Read the model definition and answer for the solid it produces. Units are mm, in the model's axes. A direction names the side the tool comes from. Coordinates: 2 decimals unless noted, no trailing zeros. Loops run counter-clockwise (first coordinate to the right, second up) from the corner with the lowest first, then second, coordinate; pieces in that order, holes last.
from build123d import *

# Parameters (mm, degrees)
SKETCH_1_R           = 2
EXTRUDE_1_DEPTH      = 16
EXTRUDE_2_DEPTH      = 3.175
SKETCH_4_R           = 3.15
CUT_EXTRUDE_6_DEPTH  = 2.775
FILLET_3_R           = 0.6
SKETCH_7_R           = 3.175
EXTRUDE_3_DEPTH      = 1.4
CUT_EXTRUDE_10_DEPTH = 10
FILLET_4_R           = 0.3
CUT_EXTRUDE_11_REACH = 18
FILLET_5_R           = 1


with BuildPart() as part:
    # 草图1 → 凸台-拉伸1 (new body)
    with BuildSketch(Plane(origin=(0, 0, 0), x_dir=(1, 0, 0), z_dir=(0, 1, 0))):
        Circle(SKETCH_1_R)
    extrude(amount=EXTRUDE_1_DEPTH)

    # 草图2 → 凸台-拉伸2 (add)
    with BuildSketch(Plane.XY):
        with BuildLine():
            Line((3.175, 16), (1.070738578, 21.991208882))
            ThreePointArc((1.070738578, 21.991208882), (-6.846541908, 23.101880092), (-3.175, 16))
            Line((-3.175, 16), (3.175, 16))
        make_face()
    extrude(amount=EXTRUDE_2_DEPTH)

    # 草图4 → 切除-拉伸6 (cut)
    with BuildSketch(Plane(origin=(0, 0, 0), x_dir=(-1, 0, 0), z_dir=(0, 0, -1))):
        with Locations((3.175, 20.5)):
            Circle(SKETCH_4_R)
    extrude(amount=-CUT_EXTRUDE_6_DEPTH, mode=Mode.SUBTRACT)

    # 圆角3
    fillet_3_edges = [part.edges().sort_by_distance(p)[0] for p in [
        (-2, 0, 0),
    ]]
    fillet(fillet_3_edges, radius=FILLET_3_R)

    # 草图7 → 凸台-拉伸3 (add)
    with BuildSketch(Plane(origin=(0, 16, 0), x_dir=(1, 0, 0), z_dir=(0, 1, 0))):
        Circle(SKETCH_7_R)
    extrude(amount=-EXTRUDE_3_DEPTH)

    # 草图11 → 切除-拉伸10 (cut, through all)
    with BuildSketch(Plane.XZ.offset(-16)):
        with BuildLine():
            Line((3.175, 3.175), (3.50604204, 0.275))
            Line((3.50604204, 0.275), (3.175, 0))
            ThreePointArc((3.175, 0), (2.24506403, 2.24506403), (0, 3.175))
            Line((0, 3.175), (3.175, 3.175))
        make_face()
    extrude(amount=-CUT_EXTRUDE_10_DEPTH, mode=Mode.SUBTRACT)

    # 草图12 → 旋转1 (revolve)
    with BuildSketch(Plane(origin=(0, 20.5, 0), x_dir=(-1, 0, 0), z_dir=(0, -1, 0))):
        with BuildLine():
            Line((3.8375, -3.175), (3.8375, -3.475))
            ThreePointArc((3.8375, -3.475), (5.765394552, -3.441974066), (7.675, -3.175))
            Line((7.675, -3.175), (3.8375, -3.175))
        make_face()
    revolve(axis=Axis((-3.8375, 20.5, 3.175), (0, 0, 1)))

    # 圆角4
    fillet_4_edges = [part.edges().sort_by_distance(p)[0] for p in [
        (-0.025, 20.5, 0),
    ]]
    fillet(fillet_4_edges, radius=FILLET_4_R)

    # 草图13 → 切除-拉伸11 (cut, up to next)
    with BuildSketch(Plane(origin=(0, 16, 0), x_dir=(1, 0, 0), z_dir=(0, 1, 0)), mode=Mode.PRIVATE) as cut_extrude_11_sk1:
        with BuildLine():
            Line((-1.4, 0), (1.4, 0))
            ThreePointArc((1.4, 0), (0, 1.4), (-1.4, 0))
        make_face()
    cut_extrude_11_tool1 = extrude(cut_extrude_11_sk1.sketch, amount=-CUT_EXTRUDE_11_REACH, mode=Mode.PRIVATE) & part.part
    add(cut_extrude_11_tool1.solids().sort_by_distance((0, 16, -0.594178))[0], mode=Mode.SUBTRACT)

    # 圆角5
    fillet_5_edges = [part.edges().sort_by_distance(p)[0] for p in [
        (0, 16, -1.4),
    ]]
    fillet(fillet_5_edges, radius=FILLET_5_R)


solid = part.part
Q1. Flat-ended cylindrical pins translate along their axes: pin 1 Ø2.5 at (x, y) = (-5.5, 18.5) entering from +Z; pin 2 Ø1 at (x, z) = (-5.5, 1) entering from -Y; pin 3 Ø1.6 at (x, z) = (1, -1) entering from +Y. Find the tip coordinate at first contact, or state that the pin passes through.
Findings below:
pin 1: stops at z = 3.48
pin 2: stops at y = 16.39
pin 3: stops at y = 15.98
Q2. Straight lines are drawn through the part: probe 1 along Y at (x, z) = (-2, -1.25); probe 2 along Y at (x, z) = (-5, 0.25); probe 3 along Z at (x, y) = (0, 1.5). For each, find the intervals that lie inside material, in ascending order.
Findings below:
probe 1: y = 14.6 to 16
probe 2: y = 16.39 to 17.93, 23.07 to 24.61
probe 3: z = -2 to -1.4, 0 to 2
Q3. A cutting plane is placed at A-A (y = 12.5). Give the vertices of the cut face in (x, z).
Findings below:
outline: circle Ø4 at (0, 0); hole (-1.4, 0) arc R1.4 ccw to (1.4, 0) - close
Q4. Which of the six approach directions +Z, -Z, +X, -X, +Y, -Y give full straight-line access (tool end or side, diameter ignored) to faces 4 (the face through (0, 7.6, -1.4)), 5 (the face through (-2.4, 24.3, 3.175)), 6 (the face through (0, 8, 2))?
Findings below:
face 4: +Y, -Y
face 5: +Z, +Y
face 6: -Y
Q5. Determine the mould class of faces 1 (the face through (1, 14.6, 2)), 2 (the face through (-1, 13, 0)), 3 (the face through (-3, 21, 2.775)) for opening direction Z: +Z half, -Z half, draft (parallel to the pull), parting line (faces both ways), or undercut.
Findings below:
face 1: draft
face 2: undercut
face 3: -Z half
